```python
from build123d import *

# Parameters (mm, degrees)
SKETCH_1_R          = 40
EXTRUDE_1_DEPTH     = 5
SKETCH_3_R          = 15
CUT_EXTRUDE_1_DEPTH = 10
SKETCH_4_R          = 2
CUT_EXTRUDE_2_DEPTH = 10
EXTRUDE_2_DEPTH     = 15
FILLET_1_R          = 10


with BuildPart() as part:
    # 草图1 → 凸台-拉伸1 (new body)
    with BuildSketch(Plane.XY):
        Circle(SKETCH_1_R)
    extrude(amount=EXTRUDE_1_DEPTH)

    # 草图3 → 切除-拉伸1 (cut)
    with BuildSketch(Plane.XY.offset(5)):
        Circle(SKETCH_3_R)
    extrude(amount=-CUT_EXTRUDE_1_DEPTH, mode=Mode.SUBTRACT)

    # 草图4 → 切除-拉伸2 (cut)
    with BuildSketch(Plane.XY.offset(5)):
        with Locations((0, -32.5)):
            Circle(SKETCH_4_R)
        with Locations((32.5, 0)):
            Circle(SKETCH_4_R)
        with Locations((-32.5, 0)):
            Circle(SKETCH_4_R)
    extrude(amount=-CUT_EXTRUDE_2_DEPTH, mode=Mode.SUBTRACT)

    # 草图5 → 凸台-拉伸2 (add)
    with BuildSketch(Plane.XY.offset(5)):
        with BuildLine():
            Line((-3, 39.88734135), (-3, 14.696938457))
            ThreePointArc((-3, 14.696938457), (0, 15), (3, 14.696938457))
            Line((3, 14.696938457), (3, 39.88734135))
            ThreePointArc((3, 39.88734135), (0, 40), (-3, 39.88734135))
        make_face()
    extrude(amount=EXTRUDE_2_DEPTH)

    # 圆角1
    fillet_1_edges = [part.edges().sort_by_distance(p)[0] for p in [
        (0, 40, 20),
        (0, 15, 20),
    ]]
    fillet(fillet_1_edges, radius=FILLET_1_R)


solid = part.part
```
Model file for the job. Use its own axes, mm. Give positions to 0.01 mm unless a question says otherwise; leave off trailing zeros. Order: outer loops, then holes, each group sorted by start corner. A loop starts at its lowest first (then second) coordinate and runs counter-clockwise, first axis right, second up.
1) Saw through at C-C, the plane x = 0. Write the cut outline in (y, z), then the cut area to 3 significant figures.
2) Saw through at D-D, the plane x = -10. Write the cut outline in (y, z), then the cut area to 3 significant figures.
3) Saw through at A-A, the plane y = 0. Write the cut outline in (x, z), then the cut area to 3 significant figures.
4) Saw through at B-B, the plane z = 3. Write the cut outline in (x, y).
5) Pin check, flat tip, straight feed: pin 1 (2 mm diameter, centred on x = -15, y = -11.5, fed in from +Z). Stop position of the tip, or through.
6) Wall check: probe 1 along Y at (x, z) = (0, 1.8); probe 2 along Z at (x, y) = (-6.5, -14); probe 3 along Y at (x, z) = (-32.5, 3.45). Give the ranges that are in metal, low to high.
7) Mould opens along X. For faces 1 (the cylindrical face through (-0.434, -34.452, 2.535)), 2 (the flat face through (3, 27, 12)), 3 (the flat face through (-3, 27, 12)) say: +X half, -X half, draft (parallel to the pull), parting line (faces both ways), or undercut.
Computed:
1. outline: (-40, 0) - (-34.5, 0) - (-34.5, 5) - (-40, 5) - close; (-30.5, 0) - (-15, 0) - (-15, 5) - (-30.5, 5) - close; (15, 0) - (40, 0) - (40, 10) arc R10 ccw to (30, 20) - (25, 20) arc R10 ccw to (15, 10) - close
1. area: 562 mm2
2. outline: (-38.73, 0) - (-11.18, 0) - (-11.18, 5) - (-38.73, 5) - close; (11.18, 0) - (38.73, 0) - (38.73, 5) - (11.18, 5) - close
2. area: 275 mm2
3. outline: (-40, 0) - (-34.5, 0) - (-34.5, 5) - (-40, 5) - close; (-30.5, 0) - (-15, 0) - (-15, 5) - (-30.5, 5) - close; (15, 0) - (30.5, 0) - (30.5, 5) - (15, 5) - close; (34.5, 0) - (40, 0) - (40, 5) - (34.5, 5) - close
3. area: 210 mm2
4. outline: circle Ø80 at (0, 0); hole circle Ø4 at (-32.5, 0); hole circle Ø30 at (0, 0); hole circle Ø4 at (0, -32.5); hole circle Ø4 at (32.5, 0)
5. pin 1: stops at z = 5
6. probe 1: y = -40 to -34.5, -30.5 to -15, 15 to 40
6. probe 2: z = 0 to 5
6. probe 3: y = -23.32 to -2, 2 to 23.32
7. face 1: undercut
7. face 2: +X half
7. face 3: -X half
